The model under review builds one solid part; all positions refer to its coordinate system, in mm. A direction names the side the tool comes from. Coordinates: 2 decimals unless noted, no trailing zeros. Write each loop counter-clockwise with the first axis right and the second up, starting at its lowest first coordinate (ties: lowest second). Pieces come first, ordered by that corner, then holes.
```python
from build123d import *

# Parameters (mm, degrees)
FILLET1_R = 0.01
FILLET2_R = 0.5


with BuildPart() as part:
    # Sketch1 → Revolve1 (revolve)
    with BuildSketch(Plane.XY):
        Polygon((0, 24), (0, 0), (1.5, 0), (1.5, 18.25), (18.5, 18.25), (18.5, 19.521176082), (15.5, 19.521176082), (13.5, 22.5), (13.5, 19.521176082), (10.5, 19.521176082), (8.5, 22.5), (8.5, 19.521176082), (4, 19.521176082), (4, 24), align=None)
    revolve(axis=Axis((0, 0, 0), (1, 0, 0)))

    # Fillet1
    fillet1_edges = [part.edges().sort_by_distance(p)[0] for p in [
        (8.5, -22.5, 0),
        (13.5, -22.5, 0),
    ]]
    fillet(fillet1_edges, radius=FILLET1_R)

    # Fillet2
    fillet2_edges = [part.edges().sort_by_distance(p)[0] for p in [
        (0, -24, 0),
    ]]
    fillet(fillet2_edges, radius=FILLET2_R)


solid = part.part
```
Item 1: Take a section at D-D, the plane x = 2.75. Write out the cut boundary in (y, z), plus the area to 3 significant figures.
Solved:
outline: circle Ø48 at (0, 0); hole circle Ø36.5 at (0, 0)
area: 763 mm2
Item 2: For pin 1 (13.5 mm diameter, centred on y = -8, z = 3.5, fed in from -X); pin 2 (1.5 mm diameter, centred on x = 5.5, y = -16, fed in from -Z); pin 3 (5 mm diameter, centred on x = 3, y = 4, fed in from +Z); pin 4 (5 mm diameter, centred on x = 9.5, y = 13.5, fed in from +Z), all flat-tipped, find the tip position at first contact; note any pin that passes through.
Solved:
pin 1: stops at x = 0
pin 2: stops at z = -12.19
pin 3: stops at z = 23.95
pin 4: stops at z = 19.49
Item 3: Take a section at C-C, the plane x = 5.75. Write out the cut boundary in (y, z).
Solved:
outline: circle Ø39.04 at (0, 0); hole circle Ø36.5 at (0, 0)
Item 4: Mouldability with a two-part tool opening along X and no side actions: class faces 4 (the face through (15.376, -4.272, -19.237)), 5 (the face through (16.979, -4.232, -19.057)), 6 (the face through (4, -3.4, -19.4)) as pulls with the +X half, pulls with the -X half, needs draft (parallel to the pull), parting line crosses it, or undercut.
Solved:
face 4: pulls with the +X half
face 5: needs draft
face 6: undercut
Item 5: Machinability: for faces 1 (the face through (10.119, -3.956, -17.816)), 2 (the face through (0, 0, 0)), 3 (the face through (8.5, -17, 10)), which of the approach directions +Z, -Z, +X, -X, +Y, -Y give a long, thin tool a straight path to every point of the face, cutting with its end or side? Answer none if there is none.
Solved:
face 1: +X
face 2: +Z, -Z, -X, +Y, -Y
face 3: none
Item 6: To check wall thickness, follow line 1 along X through (y, z) = (-18, -9); line 2 along X through (y, z) = (-21, 3); line 3 along X through (y, z) = (-2.5, 12). State the ranges of each line that lie inside material, in increasing order.
Solved:
line 1: x = 0 to 4, 8.5 to 10.09, 13.5 to 15.09
line 2: x = 0 to 4, 8.5 to 9.36, 13.5 to 14.36
line 3: x = 0 to 1.5
